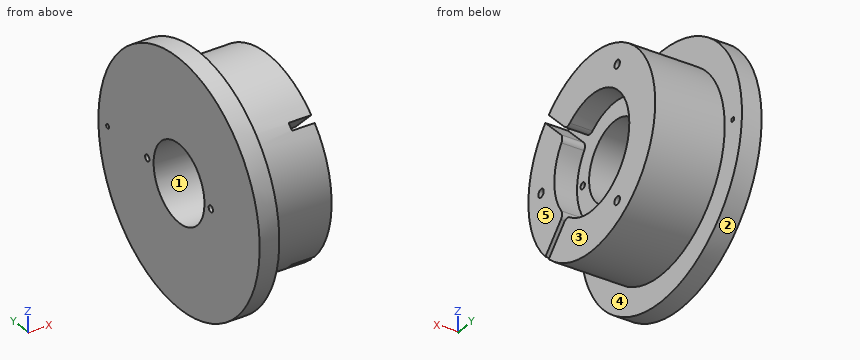
```python
from build123d import *

# Parameters (mm, degrees)
SKETCH2_R                 = 0.315
CUT_EXTRUDE1_DEPTH        = 4.4
SKETCH3_R                 = 0.425
CUT_EXTRUDE2_DEPTH        = 37.233654202
SKETCH4_R                 = 0.635
CUT_EXTRUDE3_DEPTH        = 37.018615143
FILLET1_R                 = 1.25
M2X0_4_TAPPED_HOLE1_D     = 1.6
M2X0_4_TAPPED_HOLE1_DEPTH = 7.5
M2X0_4_TAPPED_HOLE1_TIP   = 0.480688495


with BuildPart() as part:
    # Sketch1 → Revolve1 (revolve)
    with BuildSketch(Plane.XY, mode=Mode.PRIVATE) as revolve1_sk:
        Polygon((0, 23.7871), (0, 7.5), (12.872, 7.5), (12.872, 11.0635), (17.272, 11.0635), (17.272, 18.7071), (3.81, 18.7071), (3.81, 23.7871), align=None)
    revolve(revolve1_sk.sketch.rotate(Axis((12.872, 0, 0), (-1, 0, 0)), 90), axis=Axis((12.872, 0, 0), (-1, 0, 0)))

    # Sketch2 → Cut-Extrude1 (cut)
    with BuildSketch(Plane(origin=(17.272, 0, 0), x_dir=(0, 0, -1), z_dir=(1, 0, 0))):
        with BuildLine():
            Line((-0.657808531, -0.677910665), (0, 0))
            Line((0, 0), (-0.494974747, 0.494974747))
            Line((-0.494974747, 0.494974747), (-8.302376115, -7.312426621))
            ThreePointArc((-8.302376115, -7.312426621), (-7.823075874, -7.823075874), (-7.312426621, -8.302376115))
            Line((-7.312426621, -8.302376115), (-0.16558691, -1.155536403))
            Line((-0.16558691, -1.155536403), (-0.657808531, -0.677910665))
        make_face()
        with BuildLine():
            Line((-12.723678558, -13.713628052), (-7.312426621, -8.302376115))
            ThreePointArc((-7.312426621, -8.302376115), (-7.823075874, -7.823075874), (-8.302376115, -7.312426621))
            Line((-8.302376115, -7.312426621), (-13.713628052, -12.723678558))
            ThreePointArc((-13.713628052, -12.723678558), (-13.473131789, -12.978070358), (-13.227917265, -13.227917267))
            ThreePointArc((-13.227917265, -13.227917267), (-12.978070357, -13.473131789), (-12.723678558, -13.713628052))
        make_face()
        with BuildLine():
            Line((13.738626304, -12.696682153), (8.250314399, -7.371115558))
            ThreePointArc((8.250314399, -7.371115558), (7.767282545, -7.878474098), (7.253109959, -8.354246116))
            Line((7.253109959, -8.354246116), (12.750537979, -13.688658505))
            ThreePointArc((12.750537979, -13.688658505), (13.09218126, -13.362274517), (13.425472665, -13.027366354))
            ThreePointArc((13.425472665, -13.027366354), (13.58305585, -12.862977268), (13.738626304, -12.696682153))
        make_face()
        with BuildLine():
            Line((8.250314399, -7.371115558), (0.317132147, 0.326823466))
            Line((0.317132147, 0.326823466), (0, 0))
            Line((0, 0), (0.494974747, -0.494974747))
            Line((0.494974747, -0.494974747), (-0.16558691, -1.155536403))
            Line((-0.16558691, -1.155536403), (7.253109959, -8.354246116))
            ThreePointArc((7.253109959, -8.354246116), (7.767282545, -7.878474098), (8.250314399, -7.371115558))
        make_face()
        with Locations((0, -14.9775)):
            Circle(SKETCH2_R)
        with Locations((-12.970895485, 7.48875)):
            Circle(SKETCH2_R)
        with Locations((12.970895485, 7.48875)):
            Circle(SKETCH2_R)
    extrude(amount=-CUT_EXTRUDE1_DEPTH, mode=Mode.SUBTRACT)

    # Sketch3 → Cut-Extrude2 (cut, through all)
    with BuildSketch(Plane(origin=(3.81, 0, 0), x_dir=(0, 0, -1), z_dir=(1, 0, 0))):
        with Locations(Location((0, 21.082, 0), (0, 0, 90))):
            Circle(SKETCH3_R)
    extrude(amount=-CUT_EXTRUDE2_DEPTH, mode=Mode.SUBTRACT)

    # Sketch4 → Cut-Extrude3 (cut, through all)
    with BuildSketch(Plane(origin=(12.872, 0, 0), x_dir=(0, 0, -1), z_dir=(1, 0, 0))):
        with Locations(Location((0, 9.375, 0), (0, 0, 90))):
            Circle(SKETCH4_R)
        with Locations(Location((0, -9.375, 0), (0, 0, 90))):
            Circle(SKETCH4_R)
    extrude(amount=-CUT_EXTRUDE3_DEPTH, mode=Mode.SUBTRACT)

    # Fillet1
    fillet1_edges = [part.edges().sort_by_distance(p)[0] for p in [
        (15.072, -7.312426621, 8.302376115),
        (15.072, -8.302376115, 7.312426621),
        (15.072, -7.371115558, -8.250314399),
        (15.072, -8.354246116, -7.253109959),
    ]]
    fillet(fillet1_edges, radius=FILLET1_R)

    # M2x0.4 Tapped Hole1
    with Locations(Plane(origin=(17.272, 7.48875, 12.970895485), x_dir=(0, 0, 1), z_dir=(1, 0, 0))):
        with Locations((0, 0), (-25.94179097, 0), (-12.970895485, 22.46625)):
            Hole(M2X0_4_TAPPED_HOLE1_D / 2, depth=M2X0_4_TAPPED_HOLE1_DEPTH)
            with Locations((0, 0, -(M2X0_4_TAPPED_HOLE1_DEPTH + M2X0_4_TAPPED_HOLE1_TIP / 2))):  # 118° drill point
                Cone(0, M2X0_4_TAPPED_HOLE1_D / 2, M2X0_4_TAPPED_HOLE1_TIP, mode=Mode.SUBTRACT)


solid = part.part
```
Model file for the job. Use its own axes, mm. Face numbers are marked on the shaded views. A direction names the side the tool comes from. Coordinates: 2 decimals unless noted, no trailing zeros. Write each loop counter-clockwise with the first axis right and the second up, starting at its lowest first coordinate (ties: lowest second). Pieces come first, ordered by that corner, then holes. Notation, with made-up numbers: (23.5, 68) - (73.5, 68) arc R22 ccw to (73.5, 96) - close; hole circle Ø5 at (9, -31). An arc over 180 degrees is marked (long way). One line per question, with ' | ' between items. Start each with the question number.
Q1. Cut at A-A, the plane y = 0. List the corners of the cut face in (x, z), then the cut area to 3 significant figures.
Q2. Cut at C-C, the plane x = 5.25. List the corners of the cut face in (y, z) (3 decimals).
Q3. Cut at B-B, the plane x = 11.75. List the corners of the cut face in (y, z) (1 decimal).
Q4. Pin check, flat tips, straight feed: pin 1 (1.8 mm diameter, centred on y = 7.49, z = -12.97, fed in from +X); pin 2 (3 mm diameter, centred on x = 11.5, z = -3.5, fed in from -Y); pin 3 (10 mm diameter, centred on x = 10.5, y = -5.5, fed in from -Z); pin 4 (7.5 mm diameter, centred on y = -3, z = 6.5, fed in from +X). Stop position of each tip, or through.
Q5. Pull direction Y, two halves, no side cores. Call the marked faces 1, 2 and 3: pulls with the +Y half, pulls with the -Y half, needs draft (parallel to the pull), parting line crosses it, or undercut.
Q6. Drill centre lines: line 1 (Y direction, x = 14.7, z = 0); line 2 (Y direction, x = 11, z = -4.5); line 3 (X direction, y = -8.5, z = 2). Where is each one in solid material? Low to high. Write a range as [from, to].
Q7. 3-axis set-ups, long thin cutter, end or side, ignore diameter. For the marked faces 4 and 5: which of +Z, -Z, +X, -X, +Y, -Y reach the whole face in a straight line?
Q8. Cut at D-D, the plane y = 14. List the corners of the cut face in (x, z).
Answer below:
1) outline: (0, -23.79) - (3.81, -23.79) - (3.81, -18.71) - (17.27, -18.71) - (17.27, -11.06) - (12.87, -11.06) - (12.87, -7.5) - (0, -7.5) - close; (0, 7.5) - (12.87, 7.5) - (12.87, 11.06) - (17.27, 11.06) - (17.27, 18.71) - (3.81, 18.71) - (3.81, 23.79) - (0, 23.79) - close | area: 394 mm^2
2) outline: circle Ø37.414 at (0, 0); hole circle Ø1.27 at (-9.375, 0); hole circle Ø15 at (0, 0); hole circle Ø1.27 at (9.375, 0)
3) outline: circle Ø37.4 at (0, 0); hole circle Ø1.6 at (-15, 0); hole circle Ø1.3 at (-9.4, 0); hole circle Ø15 at (0, 0); hole circle Ø1.6 at (7.5, -13); hole circle Ø1.6 at (7.5, 13); hole circle Ø1.3 at (9.4, 0)
4) pin 1: x = 17.27 | pin 2: y = -18.6 | pin 3: z = -18.7 | pin 4: x = 12.87
5) face 1: undercut | face 2: parting line crosses it | face 3: needs draft
6) line 1: [-18.71, -15.78], [-14.18, -11.06], [11.06, 18.71] | line 2: [-18.16, -6], [6, 18.16] | line 3: [0, 12.87]
7) face 4: +X | face 5: +Z, -Z, +X, +Y, -Y
8) outline: (0, -19.23) - (3.81, -19.23) - (3.81, -12.41) - (17.27, -12.41) - (17.27, 12.41) - (3.81, 12.41) - (3.81, 19.23) - (0, 19.23) - close
